For this review, take the finished solid that the model builds, in its own axes (mm). A direction names the side the tool comes from. Give positions to 0.01 mm unless a question says otherwise; leave off trailing zeros. Loops run counter-clockwise (first coordinate to the right, second up) from the corner with the lowest first, then second, coordinate; pieces in that order, holes last.
```python
from build123d import *

# Parameters (mm, degrees)
BOSS_EXTRUDE1_DEPTH     = 17.78
BOSS_EXTRUDE2_START     = -0.254
BOSS_EXTRUDE2_DEPTH     = 24.638
BOSS_EXTRUDE3_START     = 328.253907246
BOSS_EXTRUDE3_OUTLINE_R = 18.542
BOSS_EXTRUDE3_DEPTH     = 84.582
CUT_EXTRUDE1_DEPTH      = 528.32
BOSS_EXTRUDE4_DEPTH     = 352.044
BOSS_EXTRUDE5_DEPTH     = 23.876


# Read off the part's stored shape, not the designer's step: Boss-Extrude3
with BuildPart() as part:
    # Sketch2 → Boss-Extrude1 (new, symmetric)
    with BuildSketch(Plane.XY):
        Polygon((60.124054664, 27.308389094), (387.937750572, 27.308389094), (387.937750572, -52.701610906), (412.835907246, -52.701610906), (412.835907246, 175.898389094), (387.937750572, 175.898389094), (387.937750572, 54.067255535), (60.124054664, 54.067255535), align=None)
    boss_extrude1 = extrude(amount=BOSS_EXTRUDE1_DEPTH, both=True)

    # 3DSketch1 → Boss-Extrude2 (add)
    with BuildSketch(Plane(origin=(387.937750572, 26.636606535, -0.300092304), x_dir=(1.1522480113550012e-15, 0.13508458090011558, -0.9908340708731408), z_dir=(1, 0, 0)).offset(BOSS_EXTRUDE2_START)):
        Polygon((0, 0), (94.376945251, -12.866806331), (96.35278288, 0), (-92.6187147, 25.763279951), (-94.376945251, 12.866806331), align=None)
    boss_extrude2 = extrude(amount=BOSS_EXTRUDE2_DEPTH)

    # Boss-Extrude3 outline → Boss-Extrude3 (add)
    with BuildSketch(Plane.YZ.offset(BOSS_EXTRUDE3_START)):
        with Locations((-52.701610906, 0)):
            Circle(BOSS_EXTRUDE3_OUTLINE_R)
    boss_extrude3 = extrude(amount=BOSS_EXTRUDE3_DEPTH)

    # 3DSketch4 → Cut-Extrude1 (cut)
    with BuildSketch(Plane(origin=(0, 190.54505023, 39.190913927), x_dir=(0, -0.6094247818041636, -0.7928438908908536), z_dir=(1, 0, 0))):
        Polygon((0, 0), (35.626268271, -46.348737362), (95.924625616, 0), (60.298357345, 46.348737362), align=None)
    cut_extrude1 = extrude(amount=CUT_EXTRUDE1_DEPTH, mode=Mode.SUBTRACT)

    # 3DSketch5 → Boss-Extrude4 (add)
    with BuildSketch(Plane(origin=(412.321750572, 39.652381829, 94.949907696), x_dir=(-2.6167454914043564e-15, 0.43787667160404403, -0.8990350496309719), z_dir=(1, 0, 0))):
        Polygon((0, 0), (12.114414059, -5.90034761), (52.872430981, 77.782771729), (40.758016921, 83.683119339), align=None)
        Polygon((171.463623123, -83.51167246), (159.39348064, -77.632887402), (200.067994044, 5.878785058), (212.138136527, 0), align=None)
    boss_extrude4 = extrude(amount=-BOSS_EXTRUDE4_DEPTH)

    # 3DSketch7 → Boss-Extrude5 (add)
    with BuildSketch(Plane(origin=(412.835907246, 127.168007467, 93.951567648), x_dir=(0, -0.42593081119403703, -0.9047557372438098), z_dir=(-1, 0, 0))):
        Polygon((0, 0), (170.799989129, -80.407313186), (173.103686862, -75.513833574), (2.303697733, 4.893479612), align=None)
        Polygon((12.745412392, 26.488926133), (183.181513062, -53.747079705), (185.685532337, -48.428080127), (15.249431667, 31.807925711), align=None)
        Polygon((24.392670249, 53.234916651), (195.324303783, -27.234370619), (198.0286446, -21.489851074), (27.097011066, 58.979436196), align=None)
        Polygon((33.959043019, 72.903233879), (205.08887574, -7.659359393), (208.694663496, 0), (37.564830775, 80.562593273), align=None)
    boss_extrude5 = extrude(amount=BOSS_EXTRUDE5_DEPTH)

    # Mirror5: Boss-Extrude1, Boss-Extrude2, Boss-Extrude3, Cut-Extrude1, Boss-Extrude4, Boss-Extrude5 across plane
    add(boss_extrude1.mirror(Plane.ZY.offset(-60.124054664)))
    add(boss_extrude2.mirror(Plane.ZY.offset(-60.124054664)))
    add(boss_extrude3.mirror(Plane.ZY.offset(-60.124054664)))
    add(cut_extrude1.mirror(Plane.ZY.offset(-60.124054664)), mode=Mode.SUBTRACT)
    add(boss_extrude4.mirror(Plane.ZY.offset(-60.124054664)))
    add(boss_extrude5.mirror(Plane.ZY.offset(-60.124054664)))


solid = part.part
```
Item 1: Take a section at D-D on x = 350. Give the boundary of the cut face in (y, z) (3 decimals), and give its area (3 significant figures).
Answer:
outline: circle Ø37.084 at (-52.702, 0); (27.308, -17.78) - (54.067, -17.78) - (54.067, 17.78) - (27.308, 17.78) - close; (39.652, -95.77) - (132.543, -95.77) - (132.543, -82.344) - (39.652, -82.344) - close; (39.652, 81.475) - (132.733, 81.475) - (132.733, 94.95) - (39.652, 94.95) - close
area: 4,530 mm2
Item 2: Take a section at C-C on y = 109. Give the boundary of the cut face in (x, z) (3 decimals), and give its area (3 significant figures).
Answer:
outline: (-292.588, -17.78) - (-267.69, -17.78) - (-267.69, 17.78) - (-292.588, 17.78) - close; (-292.074, -95.77) - (59.97, -95.77) - (59.97, -82.344) - (-292.074, -82.344) - close; (-292.074, 81.475) - (59.97, 81.475) - (59.97, 94.95) - (-292.074, 94.95) - close; (60.278, -95.77) - (412.322, -95.77) - (412.322, -82.344) - (60.278, -82.344) - close; (60.278, 81.475) - (412.322, 81.475) - (412.322, 94.95) - (60.278, 94.95) - close; (387.938, -17.78) - (412.836, -17.78) - (412.836, 17.78) - (387.938, 17.78) - close
area: 20,700 mm2
Item 3: Tool access review of faces 1 (the flat face through (328.254, -53, 0)), 2 (the flat face through (62, 53, -17.78)), 3 (the flat face through (387.938, 94, 0)): name each direction out of +Z, -Z, +X, -X, +Y, -Y from which nothing blocks a thin tool from reaching the whole face with its end or side.
Answer:
face 1: +Z, -Z, -Y
face 2: none
face 3: +Y
Item 4: For L1, parallel to Z at x = 357.5, y = 41.5 (3 decimals); L2, parallel to X at y = -22.5, z = -1.5; L3, parallel to Z at x = 322, y = 58.5 (3 decimals), list the stretches that pass through material, from the lowest coordinate up.
Answer:
L1: z = -95.77 to -82.344, -17.78 to 17.78, 81.475 to 94.95
L2: x = -292.59 to -267.69, 387.94 to 412.84
L3: z = -95.77 to -82.344, 81.475 to 94.95
Item 5: Clearance check with flat-ended pins moving along their axes: pin 1 Ø0.6 at (x, z) = (388.5, 64) entering from +Y; pin 2 Ø2 at (x, z) = (147.5, -20.5) entering from +Y; pin 3 Ø7 at (x, z) = (404, 57) entering from +Y; pin 4 Ø12 at (x, z) = (181, 7) entering from +Y. State where each tip first meets the part, or that it passes through.
Answer:
pin 1: stops at y = 39.65
pin 2: passes through
pin 3: stops at y = 127.17
pin 4: stops at y = 54.07
Item 6: Take a section at A-A on y = 10. Give the boundary of the cut face in (x, z).
Answer:
outline: (-292.59, -17.78) - (-267.69, -17.78) - (-267.69, 17.78) - (-292.59, 17.78) - close; (387.94, -17.78) - (412.84, -17.78) - (412.84, 17.78) - (387.94, 17.78) - close
Item 7: The part is to be moulded in two halves that separate along X. For faces 4 (the flat face through (239, 85, -82.344)), 5 (the flat face through (-281, 46.744, 48)), 6 (the flat face through (-267.69, -2, 0)), say which applies: released by +X, released by -X, zero draft, split by the parting line, or undercut.
Answer:
face 4: undercut
face 5: zero draft
face 6: undercut
Item 8: Take a section at B-B on x = -24.5. Give the boundary of the cut face in (y, z) (3 decimals).
Answer:
outline: (27.308, -17.78) - (54.067, -17.78) - (54.067, 17.78) - (27.308, 17.78) - close; (39.652, -95.77) - (132.543, -95.77) - (132.543, -82.344) - (39.652, -82.344) - close; (39.652, 81.475) - (132.733, 81.475) - (132.733, 94.95) - (39.652, 94.95) - close
